Here's the drawing with two shaded views (mm, measured from the low corner). I have some questions. A direction names the side the tool comes from. Coordinates: 2 decimals unless noted, no trailing zeros. Loops run counter-clockwise (first coordinate to the right, second up) from the corner with the lowest first, then second, coordinate; pieces in that order, holes last. Notation, with made-up numbers: M 3.25,-20.75 L 19.25,-20.75 A11 ccw 19.25,-8.75 Z; hole C -23.75,-8 d11. An arc over 180 degrees is marked long. Return JSON: item names as keys, results as strings. Group by question number.
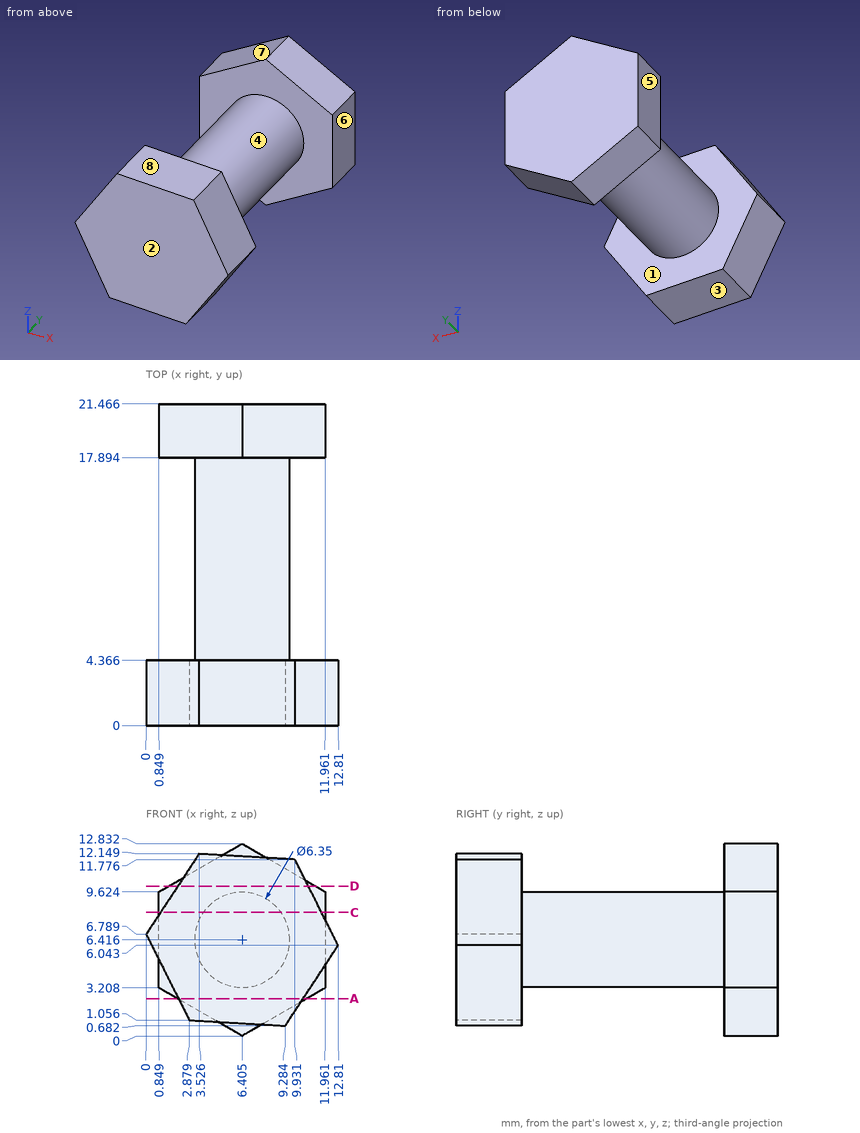
(1) We'd pull the mould along Y, two halves only. Please class the marked faces 1, 2 and 3: +Y half, -Y half, draft (parallel to the pull), parting line (faces both ways), or undercut.
(2) If I drill on L1, parallel to Y at x = 3.5, z = 3 (1 decimal); L2, parallel to X at y = 10.5, z = 7.75 (1 decimal); L3, parallel to Z at x = 6.25, y = 11.75 (1 decimal), over which ranges is the centre line in solid material (lowest first)? Write a range as [from, to].
(3) Imagine slicing it at D-D, the plane z = 10. Write out the boundary of the cut face in (x, y) (1 decimal).
(4) For the marked faces 4, 5, 6, 7 and 8, which set-ups out of +Z, -Z, +X, -X, +Y, -Y let a thin tool reach every point of the face, with its end or its side?
(5) Will these pins go through, and if not, where does the flat tip stop? P1, Ø4, axis at y = 20, z = 5.5, coming from the +X side; P2, Ø1.5, axis at y = 3, z = 1.5, coming from the -X side; P3, Ø2, axis at y = 2, z = 2.5, coming from the +X side.
(6) Imagine slicing it at C-C, the plane z = 8.25. Write out the boundary of the cut face in (x, y) (1 decimal).
(7) Imagine slicing it at A-A, the plane z = 2.5. Write out the boundary of the cut face in (x, y) (1 decimal).
Checks:
{
 "1": {"face 1": "undercut", "face 2": "-Y half", "face 3": "draft"},
 "2": {"L1": "[0, 4.4], [17.9, 21.5]", "L2": "[3.5, 9.3]", "L3": "[3.2, 9.6]"},
 "3": {"outline": "M 1.5,17.9 L 11.3,17.9 L 11.3,21.5 L 1.5,21.5 Z; M 2.1,0 L 10.8,0 L 10.8,4.4 L 2.1,4.4 Z"},
 "4": {"face 4": "none", "face 5": "+Z, -Z, -X, +Y", "face 6": "+Z, -Z, +X, +Y", "face 7": "+Z, -X, +Y", "face 8": "+Z, +X, -Y"},
 "5": {"P1": "x = 11.96", "P2": "x = 2.28", "P3": "x = 11.14"},
 "6": {"outline": "M 0.8,17.9 L 3.8,17.9 L 3.8,4.4 L 1,4.4 L 1,0 L 11.7,0 L 11.7,4.4 L 9,4.4 L 9,17.9 L 12,17.9 L 12,21.5 L 0.8,21.5 Z"},
 "7": {"outline": "M 2.1,17.9 L 10.7,17.9 L 10.7,21.5 L 2.1,21.5 Z; M 2.2,0 L 10.5,0 L 10.5,4.4 L 2.2,4.4 Z"}
}
